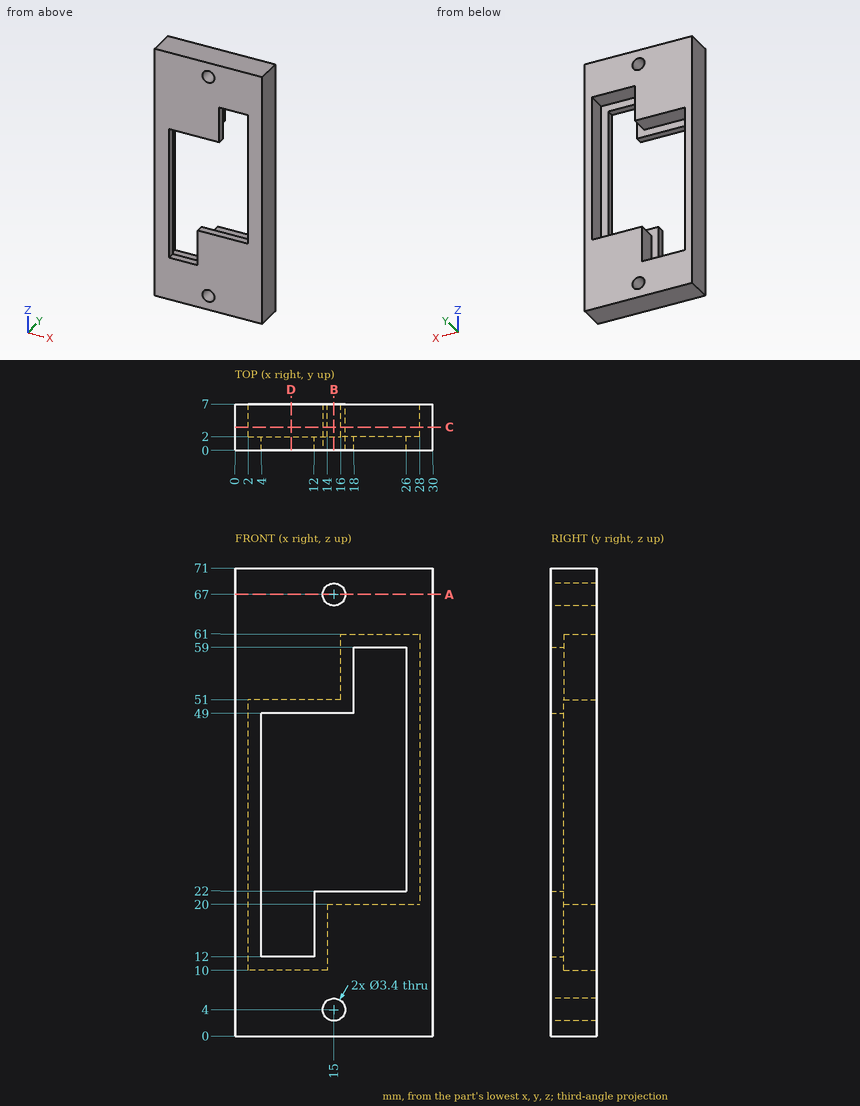
The figure shows three views and two pictorial views of one solid part (mm, origin at its lowest corner). Answer the questions. Give positions to 0.01 mm unless a question says otherwise; leave off trailing zeros. Write each loop counter-clockwise with the first axis right and the second up, starting at its lowest first coordinate (ties: lowest second). Pieces come first, ordered by that corner, then holes. Notation, with made-up numbers: (81.25, 23) - (88.25, 23) arc R24 cw to (88.25, 38) - close; hole circle Ø2 at (11, 61). An arc over 180 degrees is marked (long way). Return JSON: item names as keys, results as strings.
Q1. A cutting plane is placed at A-A, the plane z = 67. Determine the outline of the cut face in (x, y), and give its area (3 significant figures).
Reply:
{"outline": "(0, 0) - (13.3, 0) - (13.3, 7) - (0, 7) - close; (16.7, 0) - (30, 0) - (30, 7) - (16.7, 7) - close", "area": "186 mm²"}
Q2. A cutting plane is placed at C-C, the plane y = 3.5. Determine the outline of the cut face in (x, z).
Reply:
{"outline": "(0, 0) - (30, 0) - (30, 71) - (0, 71) - close; hole (2, 10) - (14, 10) - (14, 20) - (28, 20) - (28, 61) - (16, 61) - (16, 51) - (2, 51) - close; hole circle Ø3.4 at (15, 4); hole circle Ø3.4 at (15, 67)"}
Q3. A cutting plane is placed at D-D, the plane x = 8.5. Determine the outline of the cut face in (y, z), and give its area (3 significant figures).
Reply:
{"outline": "(0, 0) - (7, 0) - (7, 10) - (2, 10) - (2, 12) - (0, 12) - close; (0, 49) - (2, 49) - (2, 51) - (7, 51) - (7, 71) - (0, 71) - close", "area": "218 mm²"}
Q4. Consider line 1 along Z through (x, y) = (15, 5); line 2 along Z through (x, y) = (15, 1.75); line 3 along Z through (x, y) = (23.75, 3). Determine where each line is inside the solid, lowest interval first. Write a range as [from, to].
Reply:
{"line 1": "[0, 2.3], [5.7, 20], [51, 65.3], [68.7, 71]", "line 2": "[0, 2.3], [5.7, 22], [49, 65.3], [68.7, 71]", "line 3": "[0, 20], [61, 71]"}
Q5. Given P1, Ø13, axis at x = 16.5, z = 35, coming from the +Y side, flat-ended and moving along its own axis, determine where the tip first touches the part or whether it passes through.
Reply:
{"P1": "through"}
Q6. A cutting plane is placed at B-B, the plane x = 15. Determine the outline of the cut face in (y, z).
Reply:
{"outline": "(0, 0) - (7, 0) - (7, 2.3) - (0, 2.3) - close; (0, 5.7) - (7, 5.7) - (7, 20) - (2, 20) - (2, 22) - (0, 22) - close; (0, 49) - (2, 49) - (2, 51) - (7, 51) - (7, 65.3) - (0, 65.3) - close; (0, 68.7) - (7, 68.7) - (7, 71) - (0, 71) - close"}
